CAD build for the part. Positions are in the model's coordinates, mm. Face numbers are marked on the shaded views. Coordinates: 2 decimals unless noted, no trailing zeros. Order: outer loops, then holes, each group sorted by start corner. A loop starts at its lowest first (then second) coordinate and runs counter-clockwise, first axis right, second up.
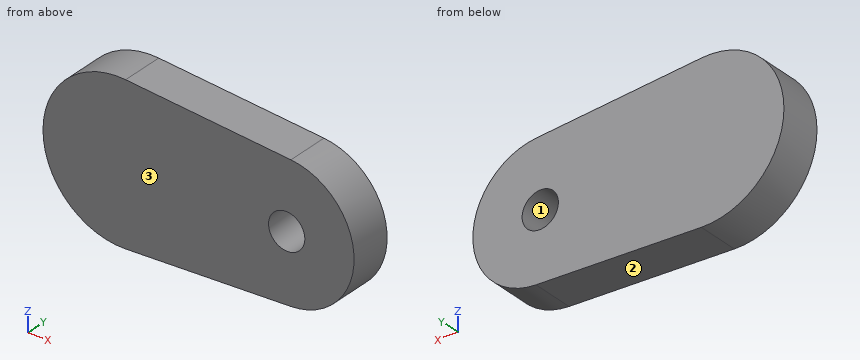
Autodesk Inventor part; units mm, degrees
ref_plane "YZ Plane" through (0, 0, 0) normal (1, 0, 0) x (0, 1, 0)
ref_plane "XZ Plane" through (0, 0, 0) normal (0, 1, 0) x (-1, 0, 0)
ref_plane "XY Plane" through (0, 0, 0) normal (0, 0, 1) x (1, 0, 0)
sketch "Sketch1" plane through (0, 0, 0) normal (0, 1, 0) x (-1, 0, 0)
  line L0 (0, 0) -> (-16, 0) construction
  line L1 (-0.4688, 7.4853) -> (-16.4063, 6.4873)
  line L2 (-16.4062, -6.4873) -> (-0.4687, -7.4853)
  arc A0 (-0.4687, -7.4853) -> (-0.4688, 7.4853) centre (0, 0) ccw
  arc A1 (-16.4063, 6.4873) -> (-16.4062, -6.4873) centre (-16, 0) ccw
  point P0 (-8, 0)
  point P1 (7.5, 0)
  point P2 (-22.5, 0)
  dimension "d0" = 7.5
  dimension "d1" = 6.5
  dimension "d2" = 30
extrude "Extrusion1" add sketch "Sketch1" along normal blind 4
hole "Hole1" at (16, 4, 0) direction (0, -1, 0) diameter 3.5 end through all
properties part number "A8-0014"
1) Slice it at A-A (z = 0). List the corners of the cut face in (x, y).
2) Drill centre lines: probe 1 along X at (y, z) = (1, 0); probe 2 along Z at (x, y) = (16, 1.75); probe 3 along Z at (x, y) = (1, 3.55). Where is each one in solid material? Low to high.
3) Two-plate mould, pull along X, no slides. Class the marked faces 1, 2 and 3: released by +X, released by -X, zero draft, split by the parting line, or undercut.
4) Pin check, flat tip, straight feed: P1, Ø1.5, axis at y = 1, z = -2.5, coming from the +X side. Stop position of the tip, or through.
5) Slice it at C-C (y = 1.4). List the corners of the cut face in (x, z), plus the area to 3 significant figures.
6) Slice it at D-D (z = -5.75). List the corners of the cut face in (x, y), plus the area to 3 significant figures.
7) Slice it at B-B (x = 16). List the corners of the cut face in (y, z).
Worked out:
1. outline: (-7.5, 0) - (14.25, 0) - (14.25, 4) - (-7.5, 4) - close; (17.75, 0) - (22.5, 0) - (22.5, 4) - (17.75, 4) - close
2. probe 1: x = -7.5 to 14.25, 17.75 to 22.5
2. probe 2: z = -6.51 to -1.75, 1.75 to 6.51
2. probe 3: z = -7.45 to 7.45
3. face 1: undercut
3. face 2: released by +X
3. face 3: zero draft
4. P1: stops at x = 22.26
5. outline: (0.47, -7.49) - (16.41, -6.49) arc R6.5 ccw to (16.41, 6.49) - (0.47, 7.49) arc R7.5 ccw (long way) to start; hole circle Ø3.5 at (16, 0)
5. area: 370 mm2
6. outline: (-4.82, 0) - (19.03, 0) - (19.03, 4) - (-4.82, 4) - close
6. area: 95.4 mm2
7. outline: (0, -6.51) - (4, -6.51) - (4, -1.75) - (0, -1.75) - close; (0, 1.75) - (4, 1.75) - (4, 6.51) - (0, 6.51) - close
